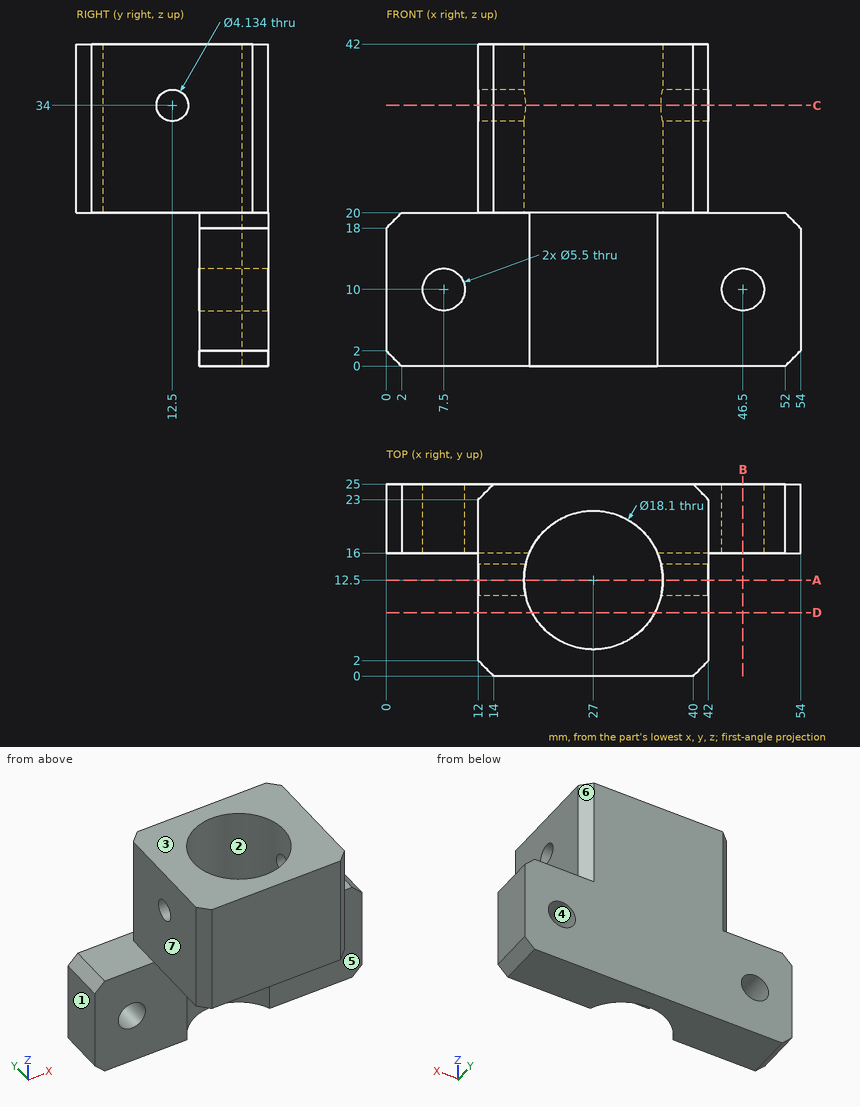
Design review of the part shown in the three views and the two pictorial views. Dimensions are in mm from the part's minimum x, y and z. A direction names the side the tool comes from. Give positions to 0.01 mm unless a question says otherwise; leave off trailing zeros. Loops run counter-clockwise (first coordinate to the right, second up) from the corner with the lowest first, then second, coordinate; pieces in that order, holes last. Notation, with made-up numbers: M 71.25,50.25 L 105.25,50.25 A25 cw 105.25,71.25 Z; hole C 53.25,81 d5. An arc over 180 degrees is marked long. Answer as a JSON object with one key per item and string values. Group by question number.
Q1. For probe 1 along X at (y, z) = (22.5, 10); probe 2 along Z at (x, y) = (46.5, 18.75); probe 3 along Z at (x, y) = (15, 12.5), list the stretches that pass through material, from the lowest coordinate up. Write a range as [from, to].
Q2. Mouldability with a two-part tool opening along X and no side actions: class the marked faces 1, 2, 3 and 4 as +X half, -X half, draft (parallel to the pull), parting line (faces both ways), or undercut.
Q3. Add section A-A on y = 12.5. Give the boundary of the cut face in (x, z), and give its area (3 significant figures).
Q4. Add section C-C on z = 34. Give the boundary of the cut face in (x, y), and give its area (3 significant figures).
Q5. Insertion check: P1, Ø10.5, axis at y = 15.5, z = 27.5, coming from the +X side; P2, Ø5.5, axis at x = 8, z = 12, coming from the -Y side; P3, Ø10, axis at y = 10, z = 9.5, coming from the +X side; P4, Ø4.5, axis at x = 7, y = 20, coming from the +Z side. Each pin has a flat end and moves straight along its axis. Give the tip position at first contact, or say it passes through.
Q6. Add section D-D on y = 8.25. Give the boundary of the cut face in (x, z), and give its area (3 significant figures).
Q7. Tool access review of the marked faces 5, 6 and 7: name each direction out of +Z, -Z, +X, -X, +Y, -Y from which nothing blocks a thin tool from reaching the whole face with its end or side.
Q8. Add section B-B on x = 46.5. Give the boundary of the cut face in (y, z), and give its area (4 significant figures).
Checked values:
{
 "1": {"probe 1": "[0, 4.75], [10.25, 43.75], [49.25, 54]", "probe 2": "[0, 7.25], [12.75, 20]", "probe 3": "[20, 31.93], [36.07, 42]"},
 "2": {"face 1": "-X half", "face 2": "undercut", "face 3": "draft", "face 4": "undercut"},
 "3": {"outline": "M 12,20 L 17.95,20 L 17.95,31.93 L 12,31.93 Z; M 12,36.07 L 17.95,36.07 L 17.95,42 L 12,42 Z; M 36.05,20 L 42,20 L 42,31.93 L 36.05,31.93 Z; M 36.05,36.07 L 42,36.07 L 42,42 L 36.05,42 Z", "area": "213 mm²"},
 "4": {"outline": "M 12,2 L 14,0 L 40,0 L 42,2 L 42,10.43 L 35.81,10.43 A9.05 cw 18.19,10.43 L 12,10.43 Z; M 12,14.57 L 18.19,14.57 A9.05 cw 35.81,14.57 L 42,14.57 L 42,23 L 40,25 L 14,25 L 12,23 Z", "area": "435 mm²"},
 "5": {"P1": "x = 42", "P2": "y = 16", "P3": "through", "P4": "z = 20"},
 "6": {"outline": "M 12,20 L 19.01,20 L 19.01,42 L 12,42 Z; M 34.99,20 L 42,20 L 42,42 L 34.99,42 Z", "area": "308 mm²"},
 "7": {"face 5": "-Z, +X, -X, -Y", "face 6": "+Z, +X, +Y", "face 7": "+Z, -X, +Y, -Y"},
 "8": {"outline": "M 16,0 L 25,0 L 25,7.25 L 16,7.25 Z; M 16,12.75 L 25,12.75 L 25,20 L 16,20 Z", "area": "130.5 mm²"}
}
